Check sheet for the modelled part. Datum: model origin and axes. Units: mm. A direction names the side the tool comes from. Coordinates: 2 decimals unless noted, no trailing zeros. Write each loop counter-clockwise with the first axis right and the second up, starting at its lowest first coordinate (ties: lowest second). Pieces come first, ordered by that corner, then holes. Notation, with made-up numbers: (20, 61.25) - (27, 61.25) arc R28 cw to (27, 93.25) - close; hole circle Ø9 at (78, 53). An arc over 180 degrees is marked (long way). Use one line per item in the form item = value. Start each with the question number.
1. Cross-section at A-A on y = 6.25. Record the boundary of the cut face in (x, z), then the cut area to 3 significant figures.
2. Tool access check on faces 1 (the face through (-67.5, -1, 0)), 2 (the face through (14, 3, -22.5)), 3 (the face through (-75, 13, -20.5)). Record the directions out of +Z, -Z, +X, -X, +Y, -Y that give a thin tool (end or side, any length) a straight path to the whole face; none if there is none.
3. Cross-section at D-D on x = 69. Record the boundary of the cut face in (y, z).
4. Cross-section at C-C on z = 3. Record the boundary of the cut face in (x, y), then the cut area to 3 significant figures.
5. Draft check along X on faces 4 (the face through (-75, 13, -0.5)), 5 (the face through (1, 0, 0)), 6 (the face through (78.5, 7, 0)). Enter one of: +X half, -X half, draft (parallel to the pull), parting line (faces both ways), or undercut.
6. Scan lines: line 1 along X through (y, z) = (14, 9.5); line 2 along Z through (x, y) = (-29, 2.5); line 3 along Y through (x, z) = (-0.5, 1.5). Record each from-to range of solid material in increasing order.
7. Cross-section at B-B on y = 13. Record the boundary of the cut face in (x, z).
8. Go/stop test with flat-tipped pins: pin 1 Ø1.5 at (x, z) = (36, -21.5) entering from -Y; pin 2 Ø3 at (y, z) = (10.5, -7) entering from -X; pin 3 Ø7.5 at (x, z) = (-76, -10.5) entering from +Y. Record where each tip stops, or that it passes through.
```python
from build123d import *

# Parameters (mm, degrees)
F0_W      = 7
F0_H      = 45
F0_W_2    = 4
F1_DEPTH  = 18
F2_W      = 143
F2_H      = 14
F3_DEPTH  = 55
F4_DEPTH  = 6
F5_W      = 10
F5_H      = 20
F6_DEPTH  = 25
F7_DEPTH  = 3
F9_W      = 7
F9_H      = 6
F10_DEPTH = 3


with BuildPart() as f1:
    # F0 (on Front) → F1 (new body)
    with BuildSketch(Plane.XZ):
        with Locations((71, 0)):
            Rectangle(F0_W, F0_H)
        Polygon((67.5, -22.5), (67.5, 22.5), (-67.5, 22.5), (-67.5, -22.5), (0, -22.5), align=None)
        with Locations((-71, 0)):
            Rectangle(F0_W, F0_H)
        with Locations((-76.5, 0)):
            Rectangle(F0_W_2, F0_H)
        with Locations((76.5, 0)):
            Rectangle(F0_W_2, F0_H)
    extrude(amount=-F1_DEPTH)

    # F2 (on face) → F3 (cut)
    with BuildSketch(Plane(origin=(0, 0, -22.5), x_dir=(1, 0, 0), z_dir=(0, 0, -1))):
        with Locations((0, -11)):
            Rectangle(F2_W, F2_H)
    extrude(amount=-F3_DEPTH, mode=Mode.SUBTRACT)

    # F2 (on face) → F4 (join)
    with BuildSketch(Plane(origin=(0, 0, -22.5), x_dir=(1, 0, 0), z_dir=(0, 0, -1))):
        Polygon((-74.5, -18), (-71.5, -18), (-71.5, -4), (-71.5, 0), (-78.5, 0), (-78.5, -18), align=None)
    extrude(amount=F4_DEPTH)

    # F5 (on face) → F6 (cut)
    with BuildSketch(Plane(origin=(-78.5, 0, 0), x_dir=(0, -1, 0), z_dir=(-1, 0, 0))):
        with Locations((-13, -10.5)):
            Rectangle(F5_W, F5_H)
    extrude(amount=-F6_DEPTH, mode=Mode.SUBTRACT)


with BuildPart() as f7:
    # F0 (on Front) → F7 (new body)
    with BuildSketch(Plane.XZ):
        with Locations((71, 0)):
            Rectangle(F0_W, F0_H)
        with Locations((76.5, 0)):
            Rectangle(F0_W_2, F0_H)
    extrude(amount=F7_DEPTH)


with BuildPart() as f7b:
    # F0 (on Front) → F7, piece 2 (new body)
    with BuildSketch(Plane.XZ):
        with Locations((-71, 0)):
            Rectangle(F0_W, F0_H)
        with Locations((-76.5, 0)):
            Rectangle(F0_W_2, F0_H)
    extrude(amount=F7_DEPTH)


with BuildPart() as f7_1:
    add(f7.part)

    # F8: union F1, F7b
    add(f1.part)
    add(f7b.part)

    # F9 (on face) → F10 (join)
    with BuildSketch(Plane.XZ):
        with Locations((-75, -25.5)):
            Rectangle(F9_W, F9_H)
    extrude(amount=F10_DEPTH)


solid = f7_1.part
```
Final values:
q1.outline = (-78.5, -28.5) - (-71.5, -28.5) - (-71.5, 22.5) - (-78.5, 22.5) - close; (71.5, -22.5) - (78.5, -22.5) - (78.5, 22.5) - (71.5, 22.5) - close
q1.area = 672 mm²
q2.face_1 = +Z, -Z, -Y
q2.face_2 = -Z, +X, +Y, -Y
q2.face_3 = -X, +Y
q3.outline = (-3, -22.5) - (4, -22.5) - (4, 22.5) - (-3, 22.5) - close
q4.outline = (-78.5, -3) - (-67.5, -3) - (-67.5, 0) - (67.5, 0) - (67.5, -3) - (78.5, -3) - (78.5, 18) - (71.5, 18) - (71.5, 4) - (-71.5, 4) - (-71.5, 18) - (-78.5, 18) - close
q4.area = 890 mm²
q5.face_4 = draft
q5.face_5 = undercut
q5.face_6 = +X half
q6.line_1 = -78.5 to -71.5, 71.5 to 78.5
q6.line_2 = -22.5 to 22.5
q6.line_3 = 0 to 4
q7.outline = (-78.5, -28.5) - (-71.5, -28.5) - (-71.5, -20.5) - (-78.5, -20.5) - close; (-78.5, -0.5) - (-71.5, -0.5) - (-71.5, 22.5) - (-78.5, 22.5) - close; (71.5, -22.5) - (78.5, -22.5) - (78.5, 22.5) - (71.5, 22.5) - close
q8.pin_1 = 0
q8.pin_2 = 71.5
q8.pin_3 = 8
